Part print with two shaded views. Sizes in mm from the minimum x, y, z corner. A direction names the side the tool comes from. Round coordinates to 2 decimals unless told otherwise and drop trailing zeros. Loops run counter-clockwise (first coordinate to the right, second up) from the corner with the lowest first, then second, coordinate; pieces in that order, holes last. Notation, with made-up numbers: (54, -33) - (110, -33) arc R23 ccw to (110, -1) - close; hole circle Ø3 at (64, 53.5). An arc over 180 degrees is marked (long way). Write each question's results on one line, items separated by ' | '. Start each with the question number.
(1) Flat gauge pins, fed straight in: P1, Ø2, axis at x = 63, z = 33, coming from the -Y side; P2, Ø11, axis at x = 16, z = 30, coming from the +Y side; P3, Ø9.5, axis at y = 31, z = 16.5, coming from the +X side; P4, Ø15.5, axis at y = 32.5, z = 29, coming from the -X side. Where does each tip first touch, or does it go through?
(2) Cut at D-D, the plane z = 56.5. List the corners of the cut face in (x, y), then the cut area to 3 significant figures.
(3) Cut at A-A, the plane z = 30. Give the number of separate pieces and of enclosed holes in the cut face, then the cut area to 3 significant figures.
(4) Tool access for the marked faces 1, 2, 3 and 4: list every direction of +Z, -Z, +X, -X, +Y, -Y with a clear straight run to the whole face (end or side of a thin tool).
(5) Cut at B-B, the plane x = 104. List the corners of the cut face in (y, z), then the cut area to 3 significant figures.
(6) Cut at C-C, the plane y = 5. List the corners of the cut face in (x, z).
(7) Drill centre lines: L1, parallel to Z at x = 104, y = 3.75; L2, parallel to X at y = 13, z = 54.5; L3, parallel to Y at x = 52, z = 20.5. Where is each one in solid material? Low to high.
(8) Mould opens along Z. For the marked faces 5, 6, 7 and 8 say: released by +Z, released by -Z, zero draft, split by the parting line, or undercut.
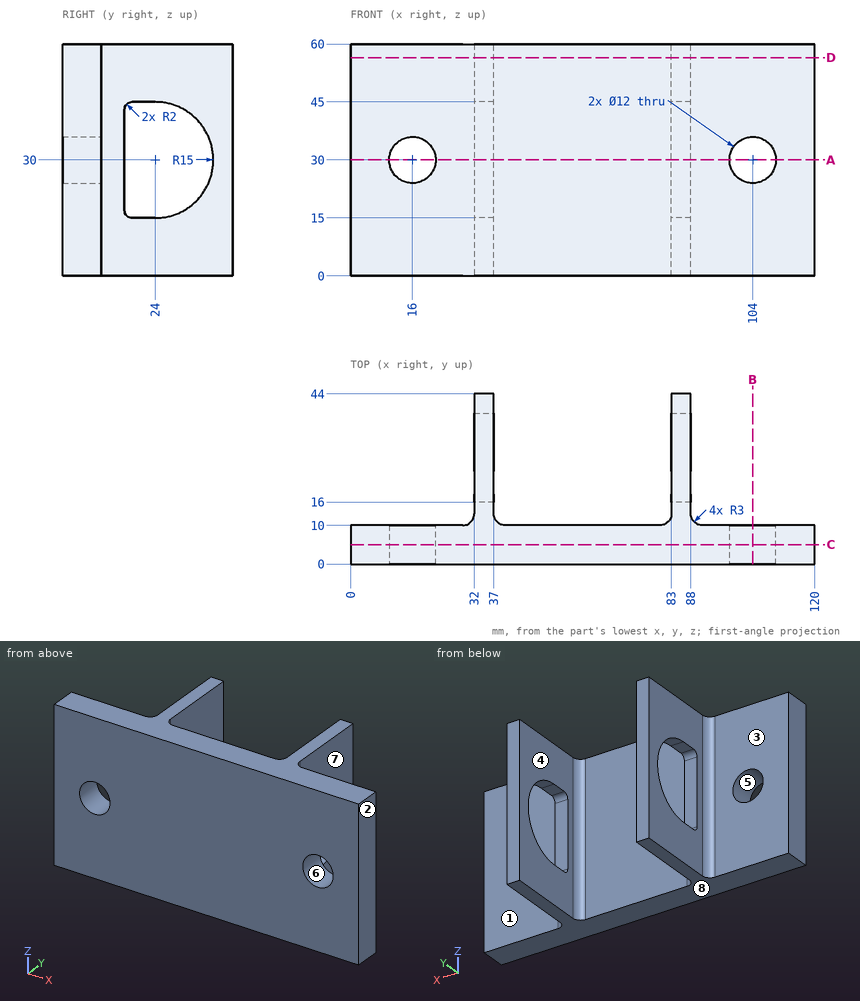
A:
1) P1: y = 0 | P2: through | P3: x = 88 | P4: x = 32
2) outline: (0, 0) - (120, 0) - (120, 10) - (91, 10) arc R3 cw to (88, 13) - (88, 44) - (83, 44) - (83, 13) arc R3 cw to (80, 10) - (40, 10) arc R3 cw to (37, 13) - (37, 44) - (32, 44) - (32, 13) arc R3 cw to (29, 10) - (0, 10) - close | area: 1,550 mm2
3) separate pieces: 5 | enclosed holes: 0 | area: 1,080 mm2
4) face 1: +Z, -Z, +X, +Y | face 2: +Z, -Z, +X, +Y, -Y | face 3: +Z, -Z, -X, +Y | face 4: +Z, -Z, +Y
5) outline: (0, 0) - (10, 0) - (10, 24) - (0, 24) - close; (0, 36) - (10, 36) - (10, 60) - (0, 60) - close | area: 480 mm2
6) outline: (0, 0) - (120, 0) - (120, 60) - (0, 60) - close; hole circle Ø12 at (16, 30); hole circle Ø12 at (104, 30)
7) L1: 0 to 24, 36 to 60 | L2: 32 to 37, 83 to 88 | L3: 0 to 10
8) face 5: undercut | face 6: undercut | face 7: zero draft | face 8: released by -Z
